Input: part model. Units: mm. Frame: model coordinates. Face numbers are marked on the shaded views. A direction names the side the tool comes from. Coordinates: 2 decimals unless noted, no trailing zeros. Loops run counter-clockwise (first coordinate to the right, second up) from the corner with the lowest first, then second, coordinate; pieces in that order, holes last. Notation, with made-up numbers: (-28.75, 0.25) - (16.25, 0.25) arc R17 cw to (16.25, 25.25) - close; hole circle Ø7 at (67.25, -22). An arc over 180 degrees is marked (long way). Answer as CSV lines item,"result". Start each with the question number.
```python
from build123d import *

# Parameters (mm, degrees)
F1_R     = 2.5
F2_DEPTH = 13
F0_R     = 4
F3_DEPTH = 5
F5_DEPTH = 3
F6_R     = 0.2


with BuildPart() as f2:
    # F1 (on face) → F2 (new body)
    with BuildSketch(Plane.XY):
        Circle(F1_R)
    extrude(amount=-F2_DEPTH)

    # F0 (on Top) → F3 (join)
    with BuildSketch(Plane.XY):
        Circle(F0_R)
    extrude(amount=-F3_DEPTH)

    # F4 (on Top) → F5 (cut)
    with BuildSketch(Plane.XY):
        Polygon((2.4999327503, -0.0183369572), (1.265846646, 2.1558367909), (-1.2340861043, 2.1741737481), (-2.4999327503, 0.0183369572), (-1.265846646, -2.1558367909), (1.2340861043, -2.1741737481), align=None)
    extrude(amount=-F5_DEPTH, mode=Mode.SUBTRACT)

    # F6
    f6_edges = [f2.edges().sort_by_distance(p)[0] for p in [
        (1.867009, -1.096255, 0),
        (-4, 0, 0),
        (1.88289, 1.06875, 0),
        (0.01588, 2.165005, 0),
        (-1.867009, 1.096255, 0),
        (-1.88289, -1.06875, 0),
        (-0.01588, -2.165005, 0),
    ]]
    fillet(f6_edges, radius=F6_R)


solid = f2.part
```
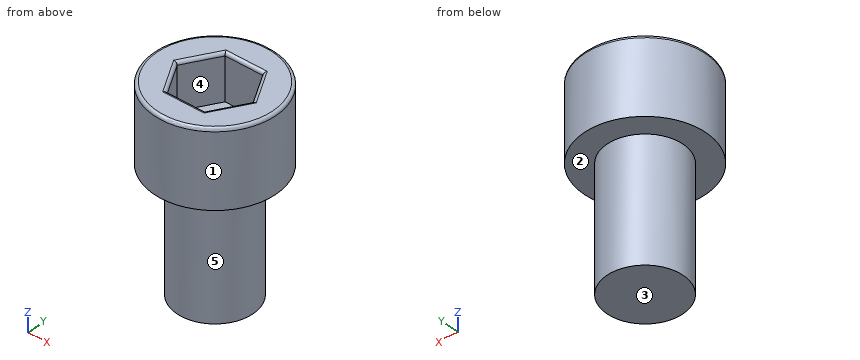
Item 1: Set-up query: the marked faces 1 and 2. Return all of +Z, -Z, +X, -X, +Y, -Y with unobstructed straight access to the full face (end or side cutting, diameter ignored); none if empty.
Item 2: Material intervals for probe 1 along Z at (x, y) = (-3.25, -0.25); probe 2 along Z at (x, y) = (-0.5, 0); probe 3 along X at (y, z) = (2, -10.75), sorted ascending.
Item 3: Contact query for flat-ended pins moving along their axis: P1, Ø4, axis at x = -3, y = 2.5, coming from the +Z side; P2, Ø2, axis at x = 2, z = -3, coming from the -Y side; P3, Ø1, axis at x = 2.5, z = -10.5, coming from the +Y side; P4, Ø1, axis at y = -1, z = -9.5, coming from the +X side. Output: stop coordinate, or through.
Item 4: Section query B-B, the plane z = -11.5. Output: boundary loops of the cut face in (x, y).
Item 5: Section query A-A, the plane z = -1. Output: boundary loops of the cut face in (x, y), and give its area (3 significant figures).
Item 6: Draft query along X for the marked faces 3, 4 and 5. Return one class per face: pulls with the +X half, pulls with the -X half, needs draft (parallel to the pull), parting line crosses it, or undercut.
Response values:
1,face 1,"+Z, -Z"
1,face 2,"-Z"
2,probe 1,"z = -5 to 0"
2,probe 2,"z = -13 to -3"
2,probe 3,"x = -1.5 to 1.5"
3,P1,"stops at z = 0"
3,P2,"stops at y = -3.87"
3,P3,"stops at y = 1.5"
3,P4,"stops at x = 2.45"
4,outline,"circle Ø5 at (0, 0)"
5,outline,"circle Ø8 at (0, 0); hole (-2.5, 0.02) - (-1.27, -2.16) - (1.23, -2.17) - (2.5, -0.02) - (1.27, 2.16) - (-1.23, 2.17) - close"
5,area,"34.0 mm²"
6,face 3,"needs draft"
6,face 4,"undercut"
6,face 5,"parting line crosses it"
